The model under review builds one solid part; all positions refer to its coordinate system, in mm. A direction names the side the tool comes from. Give positions to 0.01 mm unless a question says otherwise; leave off trailing zeros. Order: outer loops, then holes, each group sorted by start corner. A loop starts at its lowest first (then second) coordinate and runs counter-clockwise, first axis right, second up. Notation, with made-up numbers: (65.25, 52.5) - (96.25, 52.5) arc R25 cw to (96.25, 75.5) - close; hole circle Ø7 at (86.25, -40). An arc over 180 degrees is marked (long way). Write item = value, one per line. Start each with the question number.
1. Mouldability with a two-part tool opening along Z and no side actions: class faces 3 (the flat face through (4, -18.9, -24.5)), 4 (the flat face through (0, -51, -15)), 5 (the flat face through (5, -23, 0)) as pulls with the +Z half, pulls with the -Z half, needs draft (parallel to the pull), parting line crosses it, or undercut.
2. We need section D-D, the plane x = 7. Give the boundary of the cut face in (y, z), and give its area (3 significant figures).
3. For P1, Ø9, axis at y = -30.5, z = -13.5, coming from the -X side, flat-tipped, find the tip position at first contact; note if it passes through.
4. Wall thickness on probe 1 along X at (y, z) = (-9, -27.5); probe 2 along Y at (x, z) = (4.75, -10) (3 decimals); probe 3 along Y at (x, z) = (3.75, -11): over which ranges is each line inside the solid? List them lowest first.
5. We need section B-B, the plane y = -22. Give the boundary of the cut face in (x, z).
6. Machinability: for faces 1 (the cylindrical face through (5.97, -24.93, -4.48)), 2 (the cylindrical face through (1.972, -3.586, -14.615)), which of the approach directions +Z, -Z, +X, -X, +Y, -Y give a long, thin tool a straight path to every point of the face, cutting with its end or side? Answer none if there is none.
7. We need section A-A, the plane z = -22. Give the boundary of the cut face in (x, y), and give its area (3 significant figures).
8. We need section C-C, the plane x = 2.25. Give the boundary of the cut face in (y, z), and give its area (3 significant figures).
from build123d import *

# Parameters (mm, degrees)
F0_W     = 53.743943572
F0_H     = 29.5948740095
F0_R     = 10.3
F1_DEPTH = 8
F2_R     = 20
F3_DEPTH = 4
F4_DEPTH = 12.7
F5_DEPTH = 6.35


with BuildPart() as f1:
    # F0 (on Right) → F1 (new body)
    with BuildSketch(Plane.YZ):
        with Locations((-26.871971786, -14.7974370047)):
            Rectangle(F0_W, F0_H)
        with Locations((-23.5863085836, -14.6930906922)):
            Circle(F0_R, mode=Mode.SUBTRACT)
    extrude(amount=F1_DEPTH)

    # F2 (on face) → F3 (cut)
    with BuildSketch(Plane(origin=(0, 0, 0), x_dir=(0, -1, 0), z_dir=(-1, 0, 0))):
        with Locations((23.5863085836, -14.6930906922)):
            Circle(F2_R)
    extrude(amount=-F3_DEPTH, mode=Mode.SUBTRACT)

    # F4 (add): a face of the model
    f4_faces = [f1.faces().sort_by_distance(p)[0] for p in [
        (4, 0, -14.7974370047),
    ]]
    extrude(f4_faces, amount=F4_DEPTH)

    # F5 (add): a face of the model
    f5_faces = [f1.faces().sort_by_distance(p)[0] for p in [
        (4, -53.743943572, -14.7974370047),
    ]]
    extrude(f5_faces, amount=F5_DEPTH)


solid = f1.part
Model answer:
q1.face_3 = undercut
q1.face_4 = needs draft
q1.face_5 = pulls with the +Z half
q2.outline = (-60.09, -29.59) - (12.7, -29.59) - (12.7, 0) - (-60.09, 0) - close; hole circle Ø20.6 at (-23.59, -14.69)
q2.area = 1,820 mm2
q3.P1 = 4
q4.probe_1 = 4 to 8
q4.probe_2 = -60.094 to -32.755, -14.418 to 12.7
q4.probe_3 = -60.09 to -43.24, -3.93 to 12.7
q5.outline = (4, -29.59) - (8, -29.59) - (8, -24.87) - (4, -24.87) - close; (4, -4.52) - (8, -4.52) - (8, 0) - (4, 0) - close
q6.face_1 = +X, -X
q6.face_2 = -X
q7.outline = (0, -60.09) - (8, -60.09) - (8, -30.85) - (4, -30.85) - (4, -42.2) - (0, -42.2) - close; (0, -4.97) - (4, -4.97) - (4, -16.33) - (8, -16.33) - (8, 12.7) - (0, 12.7) - close
q7.area = 375 mm2
q8.outline = (-60.09, -29.59) - (-36.93, -29.59) arc R20 cw to (-37.16, 0) - (-60.09, 0) - close; (-10.25, -29.59) - (12.7, -29.59) - (12.7, 0) - (-10.02, 0) arc R20 cw to start
q8.area = 1,090 mm2
